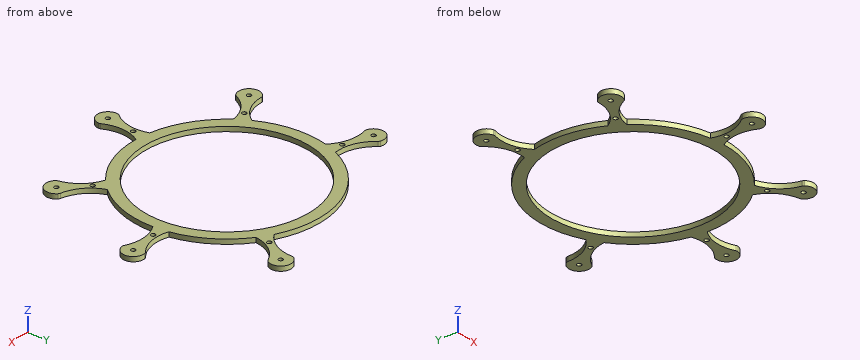
from build123d import *

# Parameters (mm, degrees)
SKETCH1_R           = 1.4605
SKETCH1_R_2         = 55.88
BOSS_EXTRUDE1_DEPTH = 3.175


with BuildPart() as part:
    # Sketch1 → Boss-Extrude1 (new body)
    with BuildSketch(Plane.XY):
        with BuildLine():
            ThreePointArc((88.371221891, 2.992104588), (75.778671602, 5.722307778), (63.466706043, 1.922066166))
            ThreePointArc((63.466706043, 1.922066166), (59.865004486, -21.176198252), (48.149108175, -41.405875631))
            ThreePointArc((48.149108175, -41.405875631), (55.331871693, -52.10275973), (66.839271225, -57.898894408))
            ThreePointArc((66.839271225, -57.898894408), (67.47896866, -58.129774903), (68.034473997, -58.522117141))
            ThreePointArc((68.034473997, -58.522117141), (68.066383731, -68.535675481), (58.053237429, -68.439394687))
            ThreePointArc((58.053237429, -68.439394687), (57.667420479, -67.877380582), (57.444971188, -67.232996469))
            ThreePointArc((57.444971188, -67.232996469), (51.728203311, -55.685490362), (41.080669811, -48.429019967))
            ThreePointArc((41.080669811, -48.429019967), (20.776095309, -60.014628604), (-2.344845215, -63.467769564))
            ThreePointArc((-2.344845215, -63.467769564), (-6.228950943, -75.752050976), (-3.586132247, -88.361783585))
            ThreePointArc((-3.586132247, -88.361783585), (-3.36770111, -89.003157809), (-3.32660045, -89.679459363))
            ThreePointArc((-3.32660045, -89.679459363), (-11.135620218, -95.947758903), (-17.303439466, -88.059135792))
            ThreePointArc((-17.303439466, -88.059135792), (-17.104674606, -87.410023107), (-16.741077367, -86.836741505))
            ThreePointArc((-16.741077367, -86.836741505), (-11.27722002, -75.167440106), (-12.242511565, -62.318527916))
            ThreePointArc((-12.242511565, -62.318527916), (-33.964407462, -53.664473517), (-51.081326085, -37.735113336))
            ThreePointArc((-51.081326085, -37.735113336), (-63.106619809, -42.363141327), (-71.313643792, -52.296473576))
            ThreePointArc((-71.313643792, -52.296473576), (-71.67843667, -52.862852869), (-72.179293677, -53.313409866))
            ThreePointArc((-72.179293677, -53.313409866), (-81.948891787, -51.116293203), (-79.626890286, -41.375621876))
            ThreePointArc((-79.626890286, -41.375621876), (-78.996252753, -41.130558358), (-78.323292008, -41.060675146))
            ThreePointArc((-78.323292008, -41.060675146), (-65.793205462, -38.056800419), (-56.34937083, -29.290939384))
            ThreePointArc((-56.34937083, -29.290939384), (-63.126842761, -6.911975648), (-61.344922052, 16.402760085))
            ThreePointArc((-61.344922052, 16.402760085), (-72.460908038, 22.91898505), (-85.344095674, 23.142163421))
            ThreePointArc((-85.344095674, 23.142163421), (-86.013413894, 23.077972745), (-86.676123345, 23.191654347))
            ThreePointArc((-86.676123345, 23.191654347), (-91.049593156, 32.199713553), (-81.986285397, 36.457508913))
            ThreePointArc((-81.986285397, 36.457508913), (-81.402337069, 36.113799392), (-80.930038908, 35.627932814))
            ThreePointArc((-80.930038908, 35.627932814), (-70.769133899, 27.704401933), (-58.027573187, 25.786339663))
            ThreePointArc((-58.027573187, 25.786339663), (-20.78382715, 59.992758023), (29.638172071, 56.145983995))
            ThreePointArc((29.638172071, 56.145983995), (38.464561255, 65.533272539), (41.548923024, 78.043789903))
            ThreePointArc((41.548923024, 78.043789903), (41.643702385, 78.713927363), (41.912089569, 79.335245044))
            ThreePointArc((41.912089569, 79.335245044), (51.667486511, 81.594581089), (53.801754345, 71.811060778))
            ThreePointArc((53.801754345, 71.811060778), (53.328466449, 71.314142081), (52.739428076, 70.96205769))
            ThreePointArc((52.739428076, 70.96205769), (42.75772259, 62.814605524), (38.058107022, 50.817562776))
            ThreePointArc((38.058107022, 50.817562776), (53.871433145, 33.600106803), (62.38288993, 11.827252681))
            ThreePointArc((62.38288993, 11.827252681), (75.225331292, 10.779382415), (86.929515737, 16.168111273))
            ThreePointArc((86.929515737, 16.168111273), (87.512909807, 16.51581617), (88.167585105, 16.696502613))
            ThreePointArc((88.167585105, 16.696502613), (96.016395661, 10.478099143), (89.698025701, 2.709536219))
            ThreePointArc((89.698025701, 2.709536219), (89.01541073, 2.76060518), (88.371221891, 2.992104588))
        make_face()
        with Locations((-10.325392041, -88.958766705)):
            Circle(SKETCH1_R, mode=Mode.SUBTRACT)
        with Locations((-8.129560177, -70.035743099)):
            Circle(SKETCH1_R, mode=Mode.SUBTRACT)
        with Locations((-75.97950865, -47.392189739)):
            Circle(SKETCH1_R, mode=Mode.SUBTRACT)
        with Locations((-59.815814277, -37.310647981)):
            Circle(SKETCH1_R, mode=Mode.SUBTRACT)
        with Locations((-84.416122315, 29.854602417)):
            Circle(SKETCH1_R, mode=Mode.SUBTRACT)
        with Locations((-66.456156975, 23.503055756)):
            Circle(SKETCH1_R, mode=Mode.SUBTRACT)
        with Locations((47.905086081, 75.649261531)):
            Circle(SKETCH1_R, mode=Mode.SUBTRACT)
        with Locations((37.716317694, 59.552942115)):
            Circle(SKETCH1_R, mode=Mode.SUBTRACT)
        with Locations((89.022339359, 9.712816136)):
            Circle(SKETCH1_R, mode=Mode.SUBTRACT)
        with Locations((70.085136904, 7.642825025)):
            Circle(SKETCH1_R, mode=Mode.SUBTRACT)
        with Locations((63.107338606, -63.544648224)):
            Circle(SKETCH1_R, mode=Mode.SUBTRACT)
        with Locations((49.68180178, -50.029565503)):
            Circle(SKETCH1_R, mode=Mode.SUBTRACT)
        with Locations((-0.003865921, -0.010935291)):
            Circle(SKETCH1_R_2, mode=Mode.SUBTRACT)
    extrude(amount=BOSS_EXTRUDE1_DEPTH)


solid = part.part
Read the model definition and answer for the solid it produces. Units are mm, in the model's axes. Round coordinates to 2 decimals unless told otherwise and drop trailing zeros. Write each loop counter-clockwise with the first axis right and the second up, starting at its lowest first coordinate (ties: lowest second). Pieces come first, ordered by that corner, then holes. Notation, with made-up numbers: (37.25, -15) - (63.25, -15) arc R15 ccw to (63.25, -5) - close; hole circle Ø11 at (60, 18). An arc over 180 degrees is marked (long way). Use a Markdown table: item, result.
(1) The part is cut by section C-C (y = 66.5). Write down the section's boundary in (x, z) (3 decimals), then the cut area to 3 significant figures.
Reported:
| item | result |
|---|---|
| outline | (38.964, 0) - (46.036, 0) - (46.036, 3.175) - (38.964, 3.175) - close |
| area | 22.5 mm2 |
(2) The part is cut by section B-B (x = -22). Write down the section's boundary in (y, z) (3 decimals).
Reported:
| item | result |
|---|---|
| outline | (-59.578, 0) - (-51.38, 0) - (-51.38, 3.175) - (-59.578, 3.175) - close; (51.358, 0) - (59.558, 0) - (59.558, 3.175) - (51.358, 3.175) - close |
(3) The part is cut by section A-A (x = -42). Write down the section's boundary in (y, z) (3 decimals).
Reported:
| item | result |
|---|---|
| outline | (-47.638, 0) - (-36.874, 0) - (-36.874, 3.175) - (-47.638, 3.175) - close; (36.852, 0) - (47.619, 0) - (47.619, 3.175) - (36.852, 3.175) - close |
(4) Straight lines are drawn through the part: line 1 along Y through (x, z) = (44.5, 2.5); line 2 along Y through (x, z) = (-8.5, 2); line 3 along X through (y, z) = (30.5, 1.45). For each, find the intervals that lie inside material, in ascending order. Write a range as [from, to].
Reported:
| item | result |
|---|---|
| line 1 | [-49.94, -33.8], [33.78, 45.28], [64.95, 81.81] |
| line 2 | [-95.75, -71.45], [-68.62, -55.24], [55.22, 62.92] |
| line 3 | [-91.42, -85.73], [-83.11, -75.68], [-55.69, -46.82], [46.81, 55.69] |
(5) Each of these flat-tipped pins is pushed along its axis until it touches: pin 1 Ø2.5 at (x, y) = (70.09, 7.64) entering from -Z; pin 2 Ø4.5 at (x, y) = (89.02, 9.71) entering from +Z (3 decimals); pin 3 Ø1.5 at (y, z) = (33.5, 0.5) entering from -X; pin 4 Ø1.5 at (x, z) = (-58.5, 2) entering from -Y. Where does it stop, or does it pass through?
Reported:
| item | result |
|---|---|
| pin 1 | through |
| pin 2 | z = 3.175 |
| pin 3 | x = -90.83 |
| pin 4 | y = -40.08 |
(6) The part is cut by section D-D (z = 2.6). State how many separate pieces and enclosed holes the cut face has, then the cut area to 3 significant figures.
Reported:
| item | result |
|---|---|
| separate pieces | 1 |
| enclosed holes | 13 |
| area | 4,420 mm2 |
